Could you check a few things on this drawing? It's one solid part, dimensions in mm from its lowest x, y, z. Round coordinates to 2 decimals unless told otherwise and drop trailing zeros. Loops run counter-clockwise (first coordinate to the right, second up) from the corner with the lowest first, then second, coordinate; pieces in that order, holes last. Notation, with made-up numbers: (-20.75, -6) -> (14.25, -6) arc R9 ccw to (14.25, 1) -> close; hole circle Ø3 at (-1.75, 37.25). An arc over 180 degrees is marked (long way). Use CSV: the item, a comma, the result in double quotes. Start each with the question number.
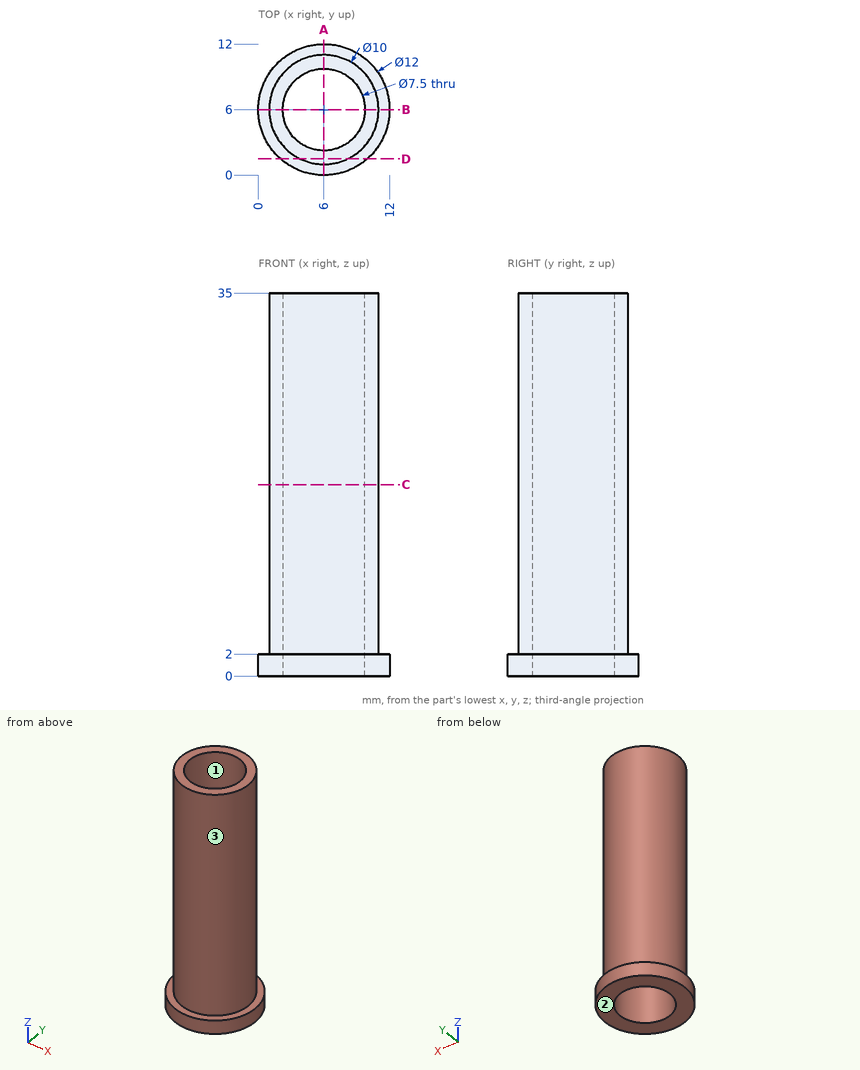
Q1. Will these pins go through, and if not, where does the flat tip stop? pin 1 Ø1.5 at (x, z) = (5.5, 27.5) entering from -Y; pin 2 Ø4 at (x, z) = (2, 15.5) entering from -Y; pin 3 Ø7 at (x, y) = (6, 6) entering from +Z; pin 4 Ø4 at (x, z) = (8.5, 7) entering from +Y.
Q2. I want a section at A-A, the plane x = 6. List the corners of the cut face in (y, z) for me.
Q3. If we mould it in two halves opening along X, with no side actions, what happens to the marked faces 1, 2 and 3? For each: pulls with the +X half, pulls with the -X half, needs draft (parallel to the pull), parting line crosses it, or undercut.
Q4. I want a section at C-C, the plane z = 17.5. List the corners of the cut face in (x, y) for me, then the cut area to 3 significant figures.
Q5. I need wall thicknesses on line 1 along X through (y, z) = (5.75, 16); line 2 along Y through (x, z) = (6, 33); line 3 along X through (y, z) = (9, 19). Which ranges of each line are inside material? Lowest first, please.
Q6. I want a section at D-D, the plane y = 1.5. List the corners of the cut face in (x, z) for me, then the cut area to 3 significant figures.
Values found:
1,pin 1,"y = 1"
1,pin 2,"y = 1.42"
1,pin 3,"through"
1,pin 4,"y = 10.97"
2,outline,"(0, 0) -> (2.25, 0) -> (2.25, 35) -> (1, 35) -> (1, 2) -> (0, 2) -> close; (9.75, 0) -> (12, 0) -> (12, 2) -> (11, 2) -> (11, 35) -> (9.75, 35) -> close"
3,face 1,"undercut"
3,face 2,"needs draft"
3,face 3,"parting line crosses it"
4,outline,"circle Ø10 at (6, 6); hole circle Ø7.5 at (6, 6)"
4,area,"34.4 mm2"
5,line 1,"1.01 to 2.26, 9.74 to 10.99"
5,line 2,"1 to 2.25, 9.75 to 11"
5,line 3,"2 to 3.75, 8.25 to 10"
6,outline,"(2.03, 0) -> (9.97, 0) -> (9.97, 2) -> (8.18, 2) -> (8.18, 35) -> (3.82, 35) -> (3.82, 2) -> (2.03, 2) -> close"
6,area,"160 mm2"
